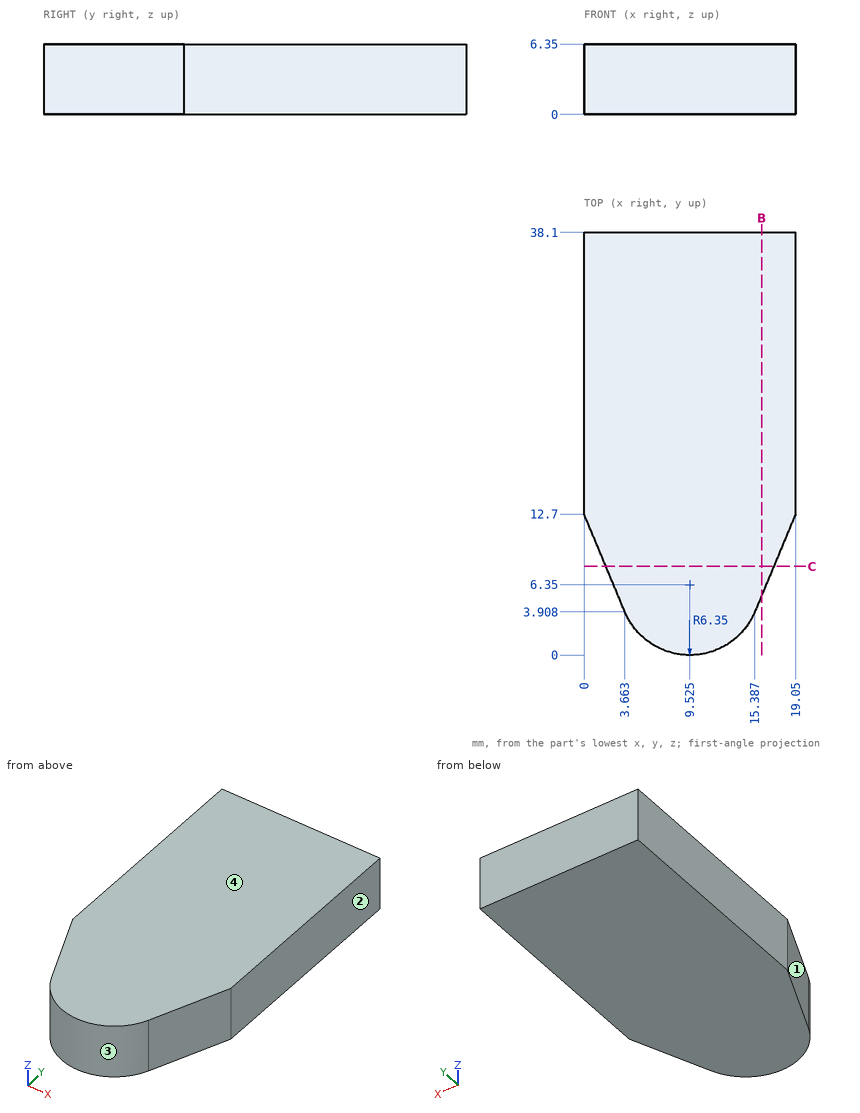
For this review, use the dimensioned drawing (mm, ordinates from the lowest corner) and the shaded views. Round coordinates to 2 decimals unless told otherwise and drop trailing zeros. Write each loop counter-clockwise with the first axis right and the second up, starting at its lowest first coordinate (ties: lowest second). Pieces come first, ordered by that corner, then holes. Notation, with made-up numbers: (-24, 27) - (32, 27) arc R21 ccw to (32, 44) - close; hole circle Ø9 at (-7, 89.25). An arc over 180 degrees is marked (long way). Answer as a JSON object with one key per item and string values.
1. We need section C-C on y = 8. Give the boundary of the cut face in (x, z).
Response values:
{"outline": "(1.96, 0) - (17.09, 0) - (17.09, 6.35) - (1.96, 6.35) - close"}
2. For pin 1 Ø6 at (x, y) = (6, 14) entering from -Z; pin 2 Ø1.5 at (x, z) = (11.5, 4.5) entering from -Y, all flat-tipped, find the tip position at first contact; note any pin that passes through.
Response values:
{"pin 1": "stops at z = 0", "pin 2": "stops at y = 0.12"}
3. Draft analysis for pull direction X (two halves, no side actions). For the marked faces 1, 2, 3 and 4, state which applies: +X half, -X half, draft (parallel to the pull), parting line (faces both ways), or undercut.
Response values:
{"face 1": "-X half", "face 2": "+X half", "face 3": "parting line", "face 4": "draft"}
4. We need section B-B on x = 16. Give the boundary of the cut face in (y, z), then the cut area to 3 significant figures.
Response values:
{"outline": "(5.38, 0) - (38.1, 0) - (38.1, 6.35) - (5.38, 6.35) - close", "area": "208 mm2"}
5. To check wall thickness, follow line 1 along Y through (x, z) = (10, 0.5); line 2 along Y through (x, z) = (3, 5.75) (1 decimal); line 3 along X through (y, z) = (11.5, 2). State the ranges of each line that lie inside material, in increasing order.
Response values:
{"line 1": "y = 0.02 to 38.1", "line 2": "y = 5.5 to 38.1", "line 3": "x = 0.5 to 18.55"}
